```python
from build123d import *

# Parameters (mm, degrees)
ESQUISSE1_W             = 100
ESQUISSE1_H             = 130
BOSS_EXTRU_1_DEPTH      = 18
ESQUISSE2_R             = 2
ENL_V_MAT_EXTRU_1_DEPTH = 204.467720042
ESQUISSE3_R             = 2
ENL_V_MAT_EXTRU_2_DEPTH = 204.467720042
ESQUISSE6_W             = 16.632413999
ESQUISSE6_H             = 56.175813279
ENL_V_MAT_EXTRU_5_DEPTH = 5
ESQUISSE8_R             = 2
ENL_V_MAT_EXTRU_6_DEPTH = 3


with BuildPart() as part:
    # Esquisse1 → Boss.-Extru.1 (new body)
    with BuildSketch(Plane(origin=(0, 0, 0), x_dir=(1, 0, 0), z_dir=(0, 1, 0))):
        with Locations((-99.482451284, -71.857991573)):
            Rectangle(ESQUISSE1_W, ESQUISSE1_H)
    extrude(amount=BOSS_EXTRU_1_DEPTH)

    # Esquisse2 → Enlèv. mat.-Extru.1 (cut, through all)
    with BuildSketch(Plane(origin=(0, 18, 0), x_dir=(1, 0, 0), z_dir=(0, 1, 0))):
        with Locations(Location((-116.573423844, -93.378684857, 0), (0, 0, 270))):
            Circle(ESQUISSE2_R)
    extrude(amount=-ENL_V_MAT_EXTRU_1_DEPTH, mode=Mode.SUBTRACT)

    # Esquisse3 → Enlèv. mat.-Extru.2 (cut, through all)
    with BuildSketch(Plane.XZ):
        with Locations(Location((-88.966331324, 52.357991573, 0), (0, 0, 270))):
            Circle(ESQUISSE3_R)
        with Locations(Location((-88.966331324, 91.357991573, 0), (0, 0, 270))):
            Circle(ESQUISSE3_R)
        with Locations(Location((-140.482451284, 91.357991573, 0), (0, 0, 270))):
            Circle(ESQUISSE3_R)
        with Locations(Location((-140.482451284, 52.357991573, 0), (0, 0, 270))):
            Circle(ESQUISSE3_R)
    extrude(amount=-ENL_V_MAT_EXTRU_2_DEPTH, mode=Mode.SUBTRACT)

    # Esquisse6 → Enlèv. mat.-Extru.5 (cut)
    with BuildSketch(Plane(origin=(0, 18, 0), x_dir=(1, 0, 0), z_dir=(0, 1, 0))):
        with Locations((-116.487794331, -71.290778218)):
            Rectangle(ESQUISSE6_W, ESQUISSE6_H)
    extrude(amount=-ENL_V_MAT_EXTRU_5_DEPTH, mode=Mode.SUBTRACT)

    # Esquisse8 → Enlèv. mat.-Extru.6 (cut)
    with BuildSketch(Plane(origin=(0, 13, 0), x_dir=(1, 0, 0), z_dir=(0, 1, 0))):
        with Locations(Location((-116.573423844, -49.202871578, 0), (0, 0, 270))):
            Circle(ESQUISSE8_R)
    extrude(amount=-ENL_V_MAT_EXTRU_6_DEPTH, mode=Mode.SUBTRACT)


solid = part.part
```
Work out the finished part from the listing and answer in its coordinate system (mm). A direction names the side the tool comes from. Coordinates: 2 decimals unless noted, no trailing zeros. Loops run counter-clockwise (first coordinate to the right, second up) from the corner with the lowest first, then second, coordinate; pieces in that order, holes last.
1) Section A-A (x = -113) is taken. Give the vertices of the cut face in (y, z).
Results:
outline: (0, 6.86) - (18, 6.86) - (18, 43.2) - (13, 43.2) - (13, 99.38) - (18, 99.38) - (18, 136.86) - (0, 136.86) - close
2) For faces 4 (the flat face through (-100, 9, 136.858)), 5 (the flat face through (-108.172, 16, 72)), determine the directions among +Z, -Z, +X, -X, +Y, -Y from which every point of the face is accessible in a straight line to the end or side of a thin tool.
Results:
face 4: +Z, +X, -X, +Y, -Y
face 5: +Y
3) Section B-B (z = 66) is taken. Give the vertices of the cut face in (x, y), plus the area to 3 significant figures.
Results:
outline: (-149.48, 0) - (-49.48, 0) - (-49.48, 18) - (-108.17, 18) - (-108.17, 13) - (-124.8, 13) - (-124.8, 18) - (-149.48, 18) - close
area: 1,720 mm2
4) Flat-ended cylindrical pins translate along their axes: pin 1 (2.5 mm diameter, centred on x = -88.97, z = 91.36, fed in from +Y); pin 2 (2 mm diameter, centred on x = -117, z = 49.5, fed in from +Y); pin 3 (5 mm diameter, centred on x = -116.57, z = 93.38, fed in from +Y). Find the tip coordinate at first contact, or state that the pin passes through.
Results:
pin 1: passes through
pin 2: stops at y = 10
pin 3: stops at y = 13
5) Consider probe 1 along X at (y, z) = (14.25, 77); probe 2 along Z at (x, y) = (-88, 14.25); probe 3 along X at (y, z) = (17.25, 93). Determine where each line is inside the solid, lowest interval first.
Results:
probe 1: x = -149.48 to -124.8, -108.17 to -49.48
probe 2: z = 6.86 to 50.61, 54.11 to 89.61, 93.11 to 136.86
probe 3: x = -149.48 to -141.62, -139.34 to -124.8, -108.17 to -90.11, -87.82 to -49.48
6) For a pull along X with two mould halves and no side action, classify faces 1 (the flat face through (-100, 9, 6.858)), 2 (the cylindrical face through (-139.13, 8.87, 92.83)), 3 (the flat face through (-149.482, 9, 73)) as +X half, -X half, draft (parallel to the pull), parting line (faces both ways), or undercut.
Results:
face 1: draft
face 2: undercut
face 3: -X half
